from build123d import *

# Parameters (mm, degrees)
BOSS_EXTRUDE1_DEPTH = 10
BOSS_EXTRUDE2_DEPTH = 10


with BuildPart() as part:
    # Sketch1 → Boss-Extrude1 (new body)
    with BuildSketch(Plane.XY):
        Polygon((127.703033666, 180.965914282), (99.942912825, 173.631948997), (96.578915919, 180.965914282), (81.052776354, 190.063780037), (72.254630601, 191.098856008), (59.316180963, 182.430094751), (60.790297203, 160.111634548), (76.653703478, 141.544593896), (63.855106266, 119.702899162), (81.052776354, 82.611392369), (102.070810081, 74.154129577), (112.205480651, 60.552230042), (143.200586682, 60.552230042), (153.335257251, 74.154129577), (174.353290979, 82.611392369), (191.550961067, 119.702899162), (178.752363855, 141.544593896), (194.61577013, 160.111634548), (196.089886369, 182.430094751), (183.151436732, 191.098856008), (174.353290979, 190.063780037), (158.827151414, 180.965914282), (155.463154508, 173.631948997), align=None)
        Polygon((67.474305777, 173.897244281), (68.387150649, 160.076562168), (79.931030202, 146.565234447), (90.026558446, 163.917673436), (90.423397797, 171.197351102), align=None, mode=Mode.SUBTRACT)
        Polygon((127.703033666, 172.577463554), (102.879615929, 166.019347867), (102.18046467, 160.076562168), (110.765700355, 126.038475421), (118.058737252, 114.76612201), (137.34733008, 114.76612201), (144.640366978, 126.038475421), (153.225602663, 160.076562168), (152.526451404, 166.019347867), align=None, mode=Mode.SUBTRACT)
        Polygon((136.586125745, 107.572158068), (118.819941588, 107.572158068), (109.172351708, 100.037547324), (109.172351708, 94.966141376), (116.6084589, 81.530126894), (138.797608433, 81.530126894), (146.233715625, 94.966141376), (146.233715625, 100.037547324), align=None, mode=Mode.SUBTRACT)
        Polygon((127.703033666, 69.222589269), (120.501208911, 66.003395505), (134.904858422, 66.003395505), align=None, mode=Mode.SUBTRACT)
        Polygon((106.298254857, 88.333075052), (112.205480651, 77.659537236), (120.314301927, 72.265301124), (113.507293972, 69.222589269), (106.298254857, 78.897953172), align=None, mode=Mode.SUBTRACT)
        Polygon((88.584904383, 87.077096627), (98.87165084, 82.611392369), (99.942912825, 93.893171548), (96.578915919, 95.353557042), align=None, mode=Mode.SUBTRACT)
        Polygon((88.013567695, 109.993210583), (91.237528294, 97.494221969), (83.484010106, 89.466752149), (72.254630601, 113.685998364), align=None, mode=Mode.SUBTRACT)
        Polygon((93.714725872, 110.641384033), (96.363799956, 100.371175761), (103.381612359, 97.324588109), (103.381612359, 103.375859749), (113.507293972, 111.283852358), (107.442428718, 119.04952661), align=None, mode=Mode.SUBTRACT)
        Polygon((72.254630601, 119.702899162), (94.729608094, 158.333436003), (103.533048595, 123.430227468), (90.476275499, 115.433025678), align=None, mode=Mode.SUBTRACT)
        Polygon((164.929791833, 115.433025678), (183.151436732, 119.702899162), (160.676459238, 158.333436003), (151.873018738, 123.430227468), align=None, mode=Mode.SUBTRACT)
        Polygon((147.963638615, 119.04952661), (161.691341461, 110.641384033), (159.042267377, 100.371175761), (152.024454974, 97.324588109), (152.024454974, 103.375859749), (141.898773361, 111.283852358), align=None, mode=Mode.SUBTRACT)
        Polygon((183.151436732, 113.685998364), (167.392499638, 109.993210583), (164.168539039, 97.494221969), (171.922057227, 89.466752149), align=None, mode=Mode.SUBTRACT)
        Polygon((158.827151414, 95.353557042), (166.821162949, 87.077096627), (156.534416493, 82.611392369), (155.463154508, 93.893171548), align=None, mode=Mode.SUBTRACT)
        Polygon((149.107812476, 78.897953172), (149.107812476, 88.333075052), (143.200586682, 77.659537236), (135.091765405, 72.265301124), (141.898773361, 69.222589269), align=None, mode=Mode.SUBTRACT)
        Polygon((164.982669535, 171.197351102), (187.931761556, 173.897244281), (187.018916684, 160.076562168), (175.475037131, 146.565234447), (165.379508887, 163.917673436), align=None, mode=Mode.SUBTRACT)
    extrude(amount=BOSS_EXTRUDE1_DEPTH)

    # Sketch2 → Boss-Extrude2 (add)
    with BuildSketch(Plane.XY.offset(10)):
        Polygon((137.703033666, 186.739416974), (127.703033666, 192.512919666), (117.703033666, 186.739416974), (117.703033666, 175.19241159), (123.949734855, 171.585876977), (127.703033666, 172.577463554), (131.456332478, 171.585876977), (137.703033666, 175.19241159), align=None)
    extrude(amount=-BOSS_EXTRUDE2_DEPTH)


solid = part.part
Input: part model. Units: mm. Frame: model coordinates. A direction names the side the tool comes from. Give positions to 0.01 mm unless a question says otherwise; leave off trailing zeros. Loops run counter-clockwise (first coordinate to the right, second up) from the corner with the lowest first, then second, coordinate; pieces in that order, holes last. Notation, with made-up numbers: (50.5, 85) -> (61.5, 85) arc R21 cw to (61.5, 91) -> close; hole circle Ø6 at (37, -1.5). An arc over 180 degrees is marked (long way). Answer as a JSON object with one key per item and string values. Group by question number.
Item 1: Pull-direction query (Y, two-part tool) for faces 1 (the flat face through (127, 113, 10)), 2 (the flat face through (107.067, 67.448, 4.93)), 3 (the flat face through (80.024, 111.865, 4.93)); classes: released by +Y, released by -Y, zero draft, split by the parting line, or undercut.
Item 2: Cut plane A-A, the plane x = 123.5. Return the cut outline in (y, z), and give its area (3 significant figures).
Item 3: Cut plane B-B, the plane y = 168. Return the cut outline in (x, z).
Item 4: Line query: probe 1 along Y at (x, z) = (173.5, 8.25); probe 2 along X at (y, z) = (156.5, 3); probe 3 along Y at (x, z) = (83.5, 5.5). Output: solid intervals per line, ascending.
Item 5: Pin query (flat end, axial travel): P1, Ø3, axis at y = 82, z = 5, coming from the -X side; P2, Ø1.8, axis at y = 101, z = 5, coming from the -X side; P3, Ø6, axis at x = 105, z = 8, coming from the +Y side. Return the tip coordinate at first contact, or that it passes through.
Item 6: Cut plane C-C, the plane z = 2.5. State how many separate pieces and enclosed holes the cut face has, and give its area (3 significant figures).
Item 7: Reachability of faces 4 (the flat face through (146.707, 175.945, 4.93)), 5 (the flat face through (185.24, 130.47, 4.93)), 6 (the flat face through (138.448, 70.765, 4.93)), 7 (the flat face through (70.344, 130.777, 4.93)) from +Z, -Z, +X, -X, +Y, -Y: full face, straight path, thin tool, end or side. Return the list, or none.
Checks:
{
 "1": {"face 1": "zero draft", "face 2": "released by -Y", "face 3": "undercut"},
 "2": {"outline": "(60.55, 0) -> (66, 0) -> (66, 10) -> (60.55, 10) -> close; (67.34, 0) -> (81.53, 0) -> (81.53, 10) -> (67.34, 10) -> close; (107.57, 0) -> (114.77, 0) -> (114.77, 10) -> (107.57, 10) -> close; (171.47, 0) -> (190.09, 0) -> (190.09, 10) -> (171.47, 10) -> close", "area": "455 mm²"},
 "3": {"outline": "(60.27, 0) -> (67.86, 0) -> (67.86, 10) -> (60.27, 10) -> close; (90.25, 0) -> (110.38, 0) -> (110.38, 10) -> (90.25, 10) -> close; (145.03, 0) -> (165.16, 0) -> (165.16, 10) -> (145.03, 10) -> close; (187.54, 0) -> (195.14, 0) -> (195.14, 10) -> (187.54, 10) -> close"},
 "4": {"probe 1": "y = 82.27 to 92.87, 111.42 to 117.44, 136.29 to 149.96, 172.2 to 189.56", "probe 2": "x = 63.88 to 71.44, 85.71 to 93.66, 95.19 to 103.08, 152.32 to 160.21, 161.74 to 169.7, 183.96 to 191.53", "probe 3": "y = 81.63 to 89.48, 111.05 to 117.07, 139.03 to 152.7, 172.01 to 188.63"},
 "5": {"P1": "stops at x = 80.64", "P2": "stops at x = 72.11", "P3": "stops at y = 175.76"},
 "6": {"separate pieces": "1", "enclosed holes": "15", "area": "6,850 mm²"},
 "7": {"face 4": "+Z, -Z, +Y", "face 5": "+Z, -Z, +X", "face 6": "+Z, -Z", "face 7": "+Z, -Z, -X"}
}
